Job drawing, mm, ordinate dimensions from the low corner. One solid piece. Give positions to 0.01 mm unless a question says otherwise; leave off trailing zeros. Write each loop counter-clockwise with the first axis right and the second up, starting at its lowest first coordinate (ties: lowest second). Pieces come first, ordered by that corner, then holes. Notation, with made-up numbers: M 1,45.5 L 45,45.5 A23 cw 45,53.5 Z; hole C -12.75,18 d1. An arc over 180 degrees is marked long. Use CSV: the item, a comma, the result in double quotes. Start each with the question number.
Item 1: Drill centre lines: line 1 (Y direction, x = 16.5, z = 1.4); line 2 (X direction, y = 19.5, z = 0.3); line 3 (X direction, y = 18.5, z = 0.35). Where is each one in solid material? Low to high. Write a range as [from, to].
Item 2: Pin check, flat tip, straight feed: pin 1 (1.5 mm diameter, centred on x = 8.5, y = 12.5, fed in from -Z). Stop position of the tip, or through.
Item 3: Cut at A-A (z = 0.5). List the corners of the cut face in (x, y), then the cut area to 3 significant figures.
Item 4: Cut at B-B (y = 5.43). List the corners of the cut face in (x, z).
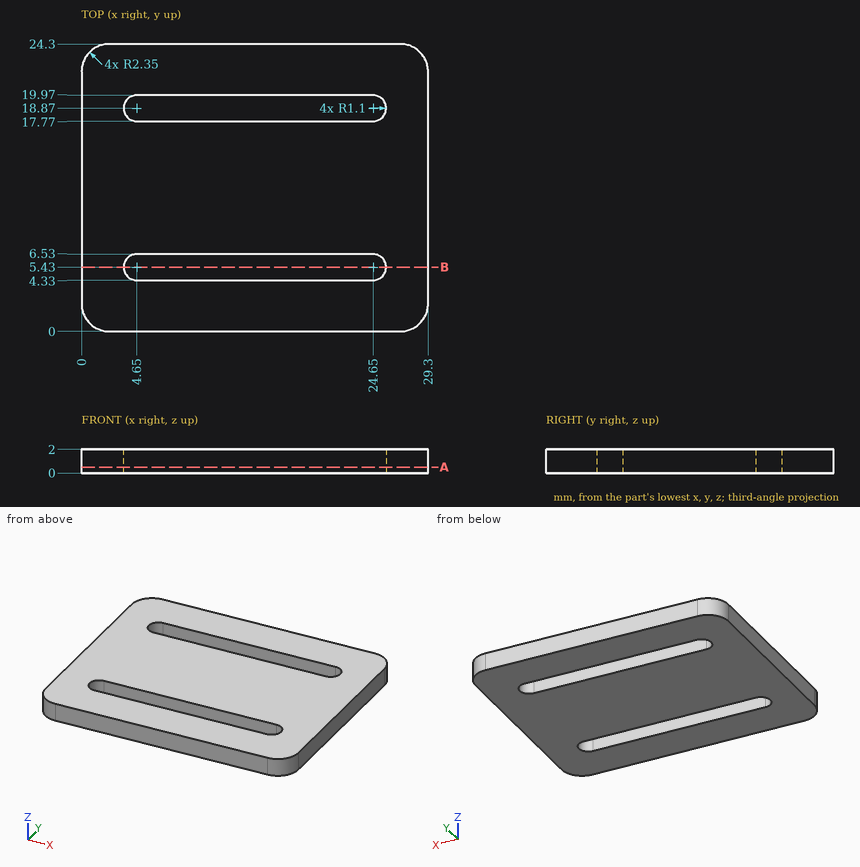
Worked answers:
1,line 1,"y = [0, 4.33], [6.53, 17.77], [19.97, 24.3]"
1,line 2,"x = [0, 3.75], [25.55, 29.3]"
1,line 3,"x = [0, 3.61], [25.69, 29.3]"
2,pin 1,"stops at z = 0"
3,outline,"M 0,2.35 A2.35 ccw 2.35,0 L 26.95,0 A2.35 ccw 29.3,2.35 L 29.3,21.95 A2.35 ccw 26.95,24.3 L 2.35,24.3 A2.35 ccw 0,21.95 Z; hole M 4.65,4.33 L 24.65,4.33 A1.1 ccw 24.65,6.53 L 4.65,6.53 A1.1 ccw Z; hole M 4.65,17.77 L 24.65,17.77 A1.1 ccw 24.65,19.97 L 4.65,19.97 A1.1 ccw Z"
3,area,"612 mm^2"
4,outline,"M 0,0 L 3.55,0 L 3.55,2 L 0,2 Z; M 25.75,0 L 29.3,0 L 29.3,2 L 25.75,2 Z"
